Could you check a few things on this model? Use its own coordinates, in mm. Face numbers are marked on the shaded views. A direction names the side the tool comes from. Coordinates: 2 decimals unless noted, no trailing zeros. Loops run counter-clockwise (first coordinate to the right, second up) from the corner with the lowest first, then second, coordinate; pieces in that order, holes last. Notation, with made-up numbers: M 30.25,-34 L 43.25,-34 A27 ccw 43.25,-17 Z; hole C 36,87 d4. An arc over 180 degrees is marked long. Return JSON: item names as keys, results as strings. Group by question number.
from build123d import *

# Parameters (mm, degrees)
SKETCH051_W       = 45
SKETCH051_H       = 20
SKETCH051_R       = 4.5
SKETCH051_R_2     = 7
PAD029_DEPTH      = 60
SKETCH052_W       = 4
SKETCH052_H       = 2
POCKET025_DEPTH   = 60.001
POCKET025_FACE1_W = 45
POCKET025_FACE1_H = 60
PAD030_DEPTH      = 20
FILLET001_R       = 3
FILLET002_R       = 2
FILLET003_R       = 2
SKETCH054_R       = 4
POCKET026_DEPTH   = 20
SKETCH053_R       = 1.75
SKETCH053_W       = 10
SKETCH053_H       = 30
SKETCH053_H_2     = 2
POCKET027_DEPTH   = 45.001


with BuildPart() as part:
    # Sketch051 → Pad029 (new body)
    with BuildSketch(Plane.XY):
        Rectangle(SKETCH051_W, SKETCH051_H)
        with Locations((-14.26955, 0)):
            Circle(SKETCH051_R, mode=Mode.SUBTRACT)
        with Locations((11.73045, 0)):
            Circle(SKETCH051_R_2, mode=Mode.SUBTRACT)
    extrude(amount=PAD029_DEPTH)

    # Sketch052 (on Face8 of Pad029) → Pocket025 (cut, through all)
    with BuildSketch(Plane.XY.offset(60)):
        with Locations((20.51, 0)):
            Rectangle(SKETCH052_W, SKETCH052_H)
    extrude(amount=-POCKET025_DEPTH, mode=Mode.SUBTRACT)

    # Pocket025 Face1 → Pad030 (add)
    with BuildSketch(Plane(origin=(0, 10, 30), x_dir=(1, 0, 0), z_dir=(0, 1, 0))):
        Rectangle(POCKET025_FACE1_W, POCKET025_FACE1_H)
    extrude(amount=PAD030_DEPTH)

    # Fillet001
    fillet001_edges = [part.edges().sort_by_distance(p)[0] for p in [
        (22.5, -10, 30),
    ]]
    fillet(fillet001_edges, radius=FILLET001_R)

    # Fillet002
    fillet002_edges = [part.edges().sort_by_distance(p)[0] for p in [
        (4.73045, 0, 60),
    ]]
    fillet(fillet002_edges, radius=FILLET002_R)

    # Fillet003
    fillet003_edges = [part.edges().sort_by_distance(p)[0] for p in [
        (4.73045, 0, 0),
    ]]
    fillet(fillet003_edges, radius=FILLET003_R)

    # Sketch054 (on Face3 of Pad030) → Pocket026 (cut)
    with BuildSketch(Plane(origin=(-22.5, 0, 0), x_dir=(0, -1, 0), z_dir=(-1, 0, 0))):
        with Locations((-20, 52.5)):
            Circle(SKETCH054_R)
        with Locations((-20, 7.5)):
            Circle(SKETCH054_R)
    extrude(amount=-POCKET026_DEPTH, mode=Mode.SUBTRACT)

    # Sketch053 (on Face15 of Pad030) → Pocket027 (cut, through all)
    with BuildSketch(Plane.YZ.offset(22.5)):
        with Locations((20, 52.5)):
            Circle(SKETCH053_R)
        with Locations((20, 7.5)):
            Circle(SKETCH053_R)
        with Locations((20, 30)):
            Rectangle(SKETCH053_W, SKETCH053_H)
        with Locations((20, 47)):
            Rectangle(SKETCH053_W, SKETCH053_H_2)
        with Locations((20, 13)):
            Rectangle(SKETCH053_W, SKETCH053_H_2)
    extrude(amount=-POCKET027_DEPTH, mode=Mode.SUBTRACT)


solid = part.part
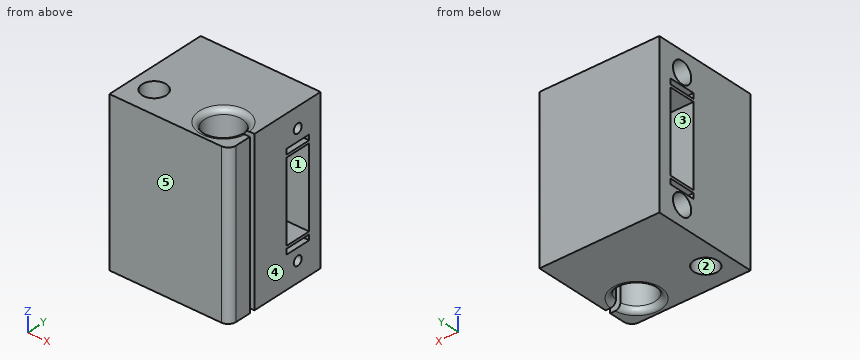
(1) Imagine slicing it at A-A, the plane z = 52.5. Write out the boundary of the cut face in (x, y), then the cut area to 3 significant figures.
(2) We'd pull the mould along Y, two halves only. Please class the marked faces 3, 4 and 5: +Y half, -Y half, draft (parallel to the pull), parting line (faces both ways), or undercut.
(3) For the marked faces 1 and 2, which set-ups out of +Z, -Z, +X, -X, +Y, -Y let a thin tool reach every point of the face, with its end or its side?
(4) If I drill on L1, parallel to Z at x = -13, y = 20; L2, parallel to Z at x = 2, y = 20; L3, parallel to Y at x = 1, z = 24, over which ranges is the centre line in solid material (lowest first)? Write a range as [from, to].
(5) Imagine slicing it at D-D, the plane y = 20. Count the separate pieces of the cut face and the enclosed holes in it, then the cut area to 3 significant figures.
(6) Imagine slicing it at C-C, the plane x = -15.5. Write out the boundary of the cut face in (y, z).
(7) Will these pins go through, and if not, where does the flat tip stop? P1, Ø5.5, axis at y = 20, z = 52.5, coming from the -X side; P2, Ø5, axis at x = 16, y = 0, coming from the -Z side.
(8) Imagine slicing it at B-B, the plane x = -5.5. Write out the boundary of the cut face in (y, z).
Checks:
{
 "1": {"outline": "M -22.5,-10 L 19.5,-10 A3 ccw 22.5,-7 L 22.5,-1 L 18.66,-1 A7 cw long 18.66,1 L 22.5,1 L 22.5,18.25 L -2.5,18.25 L -2.5,16 L -22.5,16 Z; M -22.5,24 L -2.5,24 L -2.5,21.75 L 22.5,21.75 L 22.5,30 L -22.5,30 Z; hole C -14.27,0 d9", "area": "1,330 mm²"},
 "2": {"face 3": "undercut", "face 4": "draft", "face 5": "-Y half"},
 "3": {"face 1": "+X, -X", "face 2": "+Z, -Z"},
 "4": {"L1": "[0, 3.5], [11.5, 12], [14, 15], [45, 46], [48, 48.5], [56.5, 60]", "L2": "[0, 5.75], [9.25, 12], [14, 15], [45, 46], [48, 50.75], [54.25, 60]", "L3": "[-10, 15], [25, 30]"},
 "5": {"separate pieces": "6", "enclosed holes": "0", "area": "675 mm²"},
 "6": {"outline": "M -10,0 L -4.33,0 L -4.33,60 L -10,60 Z; M 4.33,0 L 30,0 L 30,60 L 4.33,60 Z; hole M 15,12 L 25,12 L 25,14 L 15,14 Z; hole M 15,15 L 25,15 L 25,45 L 15,45 Z; hole M 15,46 L 25,46 L 25,48 L 15,48 Z; hole C 20,7.5 d8; hole C 20,52.5 d8"},
 "7": {"P1": "x = -2.5", "P2": "through"},
 "8": {"outline": "M -10,0 L 30,0 L 30,60 L -10,60 Z; hole M 15,12 L 25,12 L 25,14 L 15,14 Z; hole M 15,15 L 25,15 L 25,45 L 15,45 Z; hole M 15,46 L 25,46 L 25,48 L 15,48 Z; hole C 20,7.5 d8; hole C 20,52.5 d8"}
}
